from build123d import *

# Parameters (mm, degrees)
SKETCH_1_R          = 3
SKETCH_1_R_2        = 2
SKETCH_1_R_3        = 1.25
EXTRUDE_2_DEPTH     = 4
SKETCH_4_W          = 110
SKETCH_4_H          = 6
EXTRUDE_3_DEPTH     = 4
CUT_EXTRUDE_1_DEPTH = 4


with BuildPart() as part:
    # 草图1 → 凸台-拉伸2 (new body)
    with BuildSketch(Plane.XY):
        with BuildLine():
            Line((26.037512023, -61.503506411), (-55.962487977, -61.503506411))
            Line((-55.962487977, -61.503506411), (-55.962487977, -54.853506411))
            Line((-55.962487977, -54.853506411), (-51.962487977, -54.853506411))
            Line((-51.962487977, -54.853506411), (-51.962487977, -56.203506411))
            Line((-51.962487977, -56.203506411), (-49.262487977, -56.203506411))
            Line((-49.262487977, -56.203506411), (-49.262487977, -54.853506411))
            Line((-49.262487977, -54.853506411), (-46.562487977, -54.853506411))
            Line((-46.562487977, -54.853506411), (-46.562487977, -51.853506411))
            Line((-46.562487977, -51.853506411), (-49.262487977, -51.853506411))
            Line((-49.262487977, -51.853506411), (-49.262487977, -50.503506411))
            Line((-49.262487977, -50.503506411), (-51.962487977, -50.503506411))
            Line((-51.962487977, -50.503506411), (-51.962487977, -51.853506411))
            Line((-51.962487977, -51.853506411), (-55.962487977, -51.853506411))
            Line((-55.962487977, -51.853506411), (-55.962487977, -42.353506411))
            Line((-55.962487977, -42.353506411), (-60.962487977, -42.353506411))
            Line((-60.962487977, -42.353506411), (-60.962487977, -34.353506411))
            Line((-60.962487977, -34.353506411), (-55.962487977, -34.353506411))
            Line((-55.962487977, -34.353506411), (-55.962487977, -24.853506411))
            Line((-55.962487977, -24.853506411), (-51.962487977, -24.853506411))
            Line((-51.962487977, -24.853506411), (-51.962487977, -26.203506411))
            Line((-51.962487977, -26.203506411), (-49.262487977, -26.203506411))
            Line((-49.262487977, -26.203506411), (-49.262487977, -24.853506411))
            Line((-49.262487977, -24.853506411), (-46.562487977, -24.853506411))
            Line((-46.562487977, -24.853506411), (-46.562487977, -21.853506411))
            Line((-46.562487977, -21.853506411), (-49.262487977, -21.853506411))
            Line((-49.262487977, -21.853506411), (-49.262487977, -20.503506411))
            Line((-49.262487977, -20.503506411), (-51.962487977, -20.503506411))
            Line((-51.962487977, -20.503506411), (-51.962487977, -21.853506411))
            Line((-51.962487977, -21.853506411), (-55.962487977, -21.853506411))
            Line((-55.962487977, -21.853506411), (-55.962487977, -12.353506411))
            Line((-55.962487977, -12.353506411), (-60.962487977, -12.353506411))
            Line((-60.962487977, -12.353506411), (-60.962487977, -4.353506411))
            Line((-60.962487977, -4.353506411), (-55.962487977, -4.353506411))
            Line((-55.962487977, -4.353506411), (-55.962487977, 5.146493589))
            Line((-55.962487977, 5.146493589), (-51.962487977, 5.146493589))
            Line((-51.962487977, 5.146493589), (-51.962487977, 3.796493589))
            Line((-51.962487977, 3.796493589), (-49.262487977, 3.796493589))
            Line((-49.262487977, 3.796493589), (-49.262487977, 5.146493589))
            Line((-49.262487977, 5.146493589), (-46.562487977, 5.146493589))
            Line((-46.562487977, 5.146493589), (-46.562487977, 8.146493589))
            Line((-46.562487977, 8.146493589), (-49.262487977, 8.146493589))
            Line((-49.262487977, 8.146493589), (-49.262487977, 9.496493589))
            Line((-49.262487977, 9.496493589), (-51.962487977, 9.496493589))
            Line((-51.962487977, 9.496493589), (-51.962487977, 8.146493589))
            Line((-51.962487977, 8.146493589), (-55.962487977, 8.146493589))
            Line((-55.962487977, 8.146493589), (-55.962487977, 23.496493589))
            Line((-55.962487977, 23.496493589), (-55.962487977, 31.722989041))
            ThreePointArc((-55.962487977, 31.722989041), (-14.962487977, 51.269592797), (26.037512023, 31.722989041))
            Line((26.037512023, 31.722989041), (26.037512023, 23.496493589))
            Line((26.037512023, 23.496493589), (26.037512023, 8.146493589))
            Line((26.037512023, 8.146493589), (22.037512023, 8.146493589))
            Line((22.037512023, 8.146493589), (22.037512023, 9.496493589))
            Line((22.037512023, 9.496493589), (19.337512023, 9.496493589))
            Line((19.337512023, 9.496493589), (19.337512023, 8.146493589))
            Line((19.337512023, 8.146493589), (16.637512023, 8.146493589))
            Line((16.637512023, 8.146493589), (16.637512023, 5.146493589))
            Line((16.637512023, 5.146493589), (19.337512023, 5.146493589))
            Line((19.337512023, 5.146493589), (19.337512023, 3.796493589))
            Line((19.337512023, 3.796493589), (22.037512023, 3.796493589))
            Line((22.037512023, 3.796493589), (22.037512023, 5.146493589))
            Line((22.037512023, 5.146493589), (26.037512023, 5.146493589))
            Line((26.037512023, 5.146493589), (26.037512023, -4.353506411))
            Line((26.037512023, -4.353506411), (31.037512023, -4.353506411))
            Line((31.037512023, -4.353506411), (31.037512023, -12.353506411))
            Line((31.037512023, -12.353506411), (26.037512023, -12.353506411))
            Line((26.037512023, -12.353506411), (26.037512023, -21.853506411))
            Line((26.037512023, -21.853506411), (22.037512023, -21.853506411))
            Line((22.037512023, -21.853506411), (22.037512023, -20.503506411))
            Line((22.037512023, -20.503506411), (19.337512023, -20.503506411))
            Line((19.337512023, -20.503506411), (19.337512023, -21.853506411))
            Line((19.337512023, -21.853506411), (16.637512023, -21.853506411))
            Line((16.637512023, -21.853506411), (16.637512023, -24.853506411))
            Line((16.637512023, -24.853506411), (19.337512023, -24.853506411))
            Line((19.337512023, -24.853506411), (19.337512023, -26.203506411))
            Line((19.337512023, -26.203506411), (22.037512023, -26.203506411))
            Line((22.037512023, -26.203506411), (22.037512023, -24.853506411))
            Line((22.037512023, -24.853506411), (26.037512023, -24.853506411))
            Line((26.037512023, -24.853506411), (26.037512023, -34.353506411))
            Line((26.037512023, -34.353506411), (31.037512023, -34.353506411))
            Line((31.037512023, -34.353506411), (31.037512023, -42.353506411))
            Line((31.037512023, -42.353506411), (26.037512023, -42.353506411))
            Line((26.037512023, -42.353506411), (26.037512023, -51.853506411))
            Line((26.037512023, -51.853506411), (22.037512023, -51.853506411))
            Line((22.037512023, -51.853506411), (22.037512023, -50.503506411))
            Line((22.037512023, -50.503506411), (19.337512023, -50.503506411))
            Line((19.337512023, -50.503506411), (19.337512023, -51.853506411))
            Line((19.337512023, -51.853506411), (16.637512023, -51.853506411))
            Line((16.637512023, -51.853506411), (16.637512023, -54.853506411))
            Line((16.637512023, -54.853506411), (19.337512023, -54.853506411))
            Line((19.337512023, -54.853506411), (19.337512023, -56.203506411))
            Line((19.337512023, -56.203506411), (22.037512023, -56.203506411))
            Line((22.037512023, -56.203506411), (22.037512023, -54.853506411))
            Line((22.037512023, -54.853506411), (26.037512023, -54.853506411))
            Line((26.037512023, -54.853506411), (26.037512023, -61.503506411))
        make_face()
        with Locations((-14.962487977, -25.253506411)):
            Circle(SKETCH_1_R, mode=Mode.SUBTRACT)
        with Locations((4.523083608, -12.753506411)):
            Circle(SKETCH_1_R, mode=Mode.SUBTRACT)
        with Locations((-14.962487977, -1.503506411)):
            Circle(SKETCH_1_R_2, mode=Mode.SUBTRACT)
        with Locations((-35.530591317, 10.371493589)):
            Circle(SKETCH_1_R, mode=Mode.SUBTRACT)
        with Locations((-34.448059562, -12.753506411)):
            Circle(SKETCH_1_R, mode=Mode.SUBTRACT)
        with Locations((5.605615363, 10.371493589)):
            Circle(SKETCH_1_R, mode=Mode.SUBTRACT)
        with Locations((-14.962487977, 20.996493589)):
            Circle(SKETCH_1_R, mode=Mode.SUBTRACT)
        with Locations((18.271530739, -34.737525127)):
            Circle(SKETCH_1_R_2, mode=Mode.SUBTRACT)
        with Locations((-14.962487977, -48.503506411)):
            Circle(SKETCH_1_R_2, mode=Mode.SUBTRACT)
        with Locations((-48.196506692, -34.737525127)):
            Circle(SKETCH_1_R_2, mode=Mode.SUBTRACT)
        with Locations((-48.196506692, 31.730512305)):
            Circle(SKETCH_1_R_2, mode=Mode.SUBTRACT)
        with Locations((-14.962487977, 45.496493589)):
            Circle(SKETCH_1_R_2, mode=Mode.SUBTRACT)
        with Locations((18.271530739, 31.730512305)):
            Circle(SKETCH_1_R_2, mode=Mode.SUBTRACT)
        with Locations((-14.962487977, 7.996493589)):
            Circle(SKETCH_1_R_3, mode=Mode.SUBTRACT)
        with Locations((-5.462487977, -1.503506411)):
            Circle(SKETCH_1_R_3, mode=Mode.SUBTRACT)
        with Locations((-14.962487977, -11.003506411)):
            Circle(SKETCH_1_R_3, mode=Mode.SUBTRACT)
        with Locations((-24.462487977, -1.503506411)):
            Circle(SKETCH_1_R_3, mode=Mode.SUBTRACT)
    extrude(amount=EXTRUDE_2_DEPTH)

    # 草图4 → 凸台-拉伸3 (add)
    with BuildSketch(Plane.XY.offset(4)):
        with Locations((-14.962487977, -64.503506411)):
            Rectangle(SKETCH_4_W, SKETCH_4_H)
    extrude(amount=-EXTRUDE_3_DEPTH)

    # 草图5 → 切除-拉伸1 (cut)
    with BuildSketch(Plane.XY.offset(4)):
        Polygon((-60.962487977, -4.353506411), (-59.762487977, -4.353506411), (-60.962487977, -5.553506411), align=None)
        Polygon((-60.962487977, -12.353506411), (-59.762487977, -12.353506411), (-60.962487977, -11.153506411), align=None)
        Polygon((-60.962487977, -34.353506411), (-59.762487977, -34.353506411), (-60.962487977, -35.553506411), align=None)
        Polygon((-60.962487977, -42.353506411), (-59.762487977, -42.353506411), (-60.962487977, -41.153506411), align=None)
        Polygon((31.037512023, -42.353506411), (31.037512023, -41.153506411), (29.837512023, -42.353506411), align=None)
        Polygon((29.837512023, -34.353506411), (31.037512023, -34.353506411), (31.037512023, -35.553506411), align=None)
        Polygon((31.037512023, -12.353506411), (29.837512023, -12.353506411), (31.037512023, -11.153506411), align=None)
        Polygon((31.037512023, -4.353506411), (29.837512023, -4.353506411), (31.037512023, -5.553506411), align=None)
    extrude(amount=-CUT_EXTRUDE_1_DEPTH, mode=Mode.SUBTRACT)


solid = part.part
Verification items for the finished model (mm, model axes). A direction names the side the tool comes from. Give positions to 0.01 mm unless a question says otherwise; leave off trailing zeros. Loops run counter-clockwise (first coordinate to the right, second up) from the corner with the lowest first, then second, coordinate; pieces in that order, holes last. Notation, with made-up numbers: (9.5, 5.5) - (15.5, 5.5) arc R20 ccw to (15.5, 13.5) - close; hole circle Ø4 at (22, 26.5). An arc over 180 degrees is marked (long way). Write each question's results on one line, items separated by ' | '.
1) Sectioned sample at B-B on y = 28. Record the boundary of the cut face in (x, z), plus the area to 3 significant figures.
Solution:
outline: (-55.96, 0) - (26.04, 0) - (26.04, 4) - (-55.96, 4) - close | area: 328 mm2
2) Material ranges on L1, parallel to X at y = -51, z = 1; L2, parallel to X at y = -34.5, z = 3.3; L3, parallel to X at y = -10.5, z = 0.3, recorded low to high. Write a range as from..to.
Solution:
L1: -55.96..-51.96, -49.26..19.34, 22.04..26.04 | L2: -59.91..-50.18, -46.21..16.29, 20.26..29.98 | L3: -60.96..-36.43, -32.47..-16.11, -13.82..2.54, 6.5..31.04
3) Tool access check on faces 1 (the flat face through (-54, -21.854, 2)), 2 (the flat face through (24, 8.146, 2)), 3 (the flat face through (21, -26.204, 2)). Record the directions out of +Z, -Z, +X, -X, +Y, -Y that give a thin tool (end or side, any length) a straight path to the whole face; none if there is none.
Solution:
face 1: +Z, -Z, -X | face 2: +Z, -Z, +X | face 3: +Z, -Z
4) Sectioned sample at C-C on x = 14. Record the boundary of the cut face in (y, z).
Solution:
outline: (-67.5, 0) - (42.61, 0) - (42.61, 4) - (-67.5, 4) - close
5) Depth check by flat-ended pin: P1, Ø1.1, axis at y = -25.5, z = 2, coming from the -X side; P2, Ø1.4, axis at x = -51, z = 2, coming from the +Y side; P3, Ø1.2, axis at x = 24.5, z = 2, coming from the +Y side. Enter the tip coordinate at first touch or a pass-through.
Solution:
P1: x = -55.96 | P2: y = 37.69 | P3: y = 34.2
6) Mould release check, pull along Y, two halves, no side actions. Record for faces 4 (the flat face through (18, -24.854, 2)), 5 (the cylindrical face through (-15.62, 51.265, 1.972)), 6 (the flat face through (26.038, 0, 2)): pulls with the +Y half, pulls with the -Y half, needs draft (parallel to the pull), parting line crosses it, or undercut.
Solution:
face 4: undercut | face 5: pulls with the +Y half | face 6: needs draft
7) Sectioned sample at A-A on z = 1.8. Count the separate pieces of the cut face and the enclosed holes in it, plus the area to 3 significant figures.
Solution:
separate pieces: 1 | enclosed holes: 17 | area: 9,080 mm2
